Here's the drawing with two shaded views (mm, measured from the low corner). I have some questions. Round coordinates to 2 decimals unless told otherwise and drop trailing zeros. Loops run counter-clockwise (first coordinate to the right, second up) from the corner with the lowest first, then second, coordinate; pieces in that order, holes last. Notation, with made-up numbers: (16, -10) -> (24, -10) arc R19 ccw to (24, -3) -> close; hole circle Ø8 at (52.5, -30.5). An arc over 180 degrees is marked (long way). Write item = value, one per line.
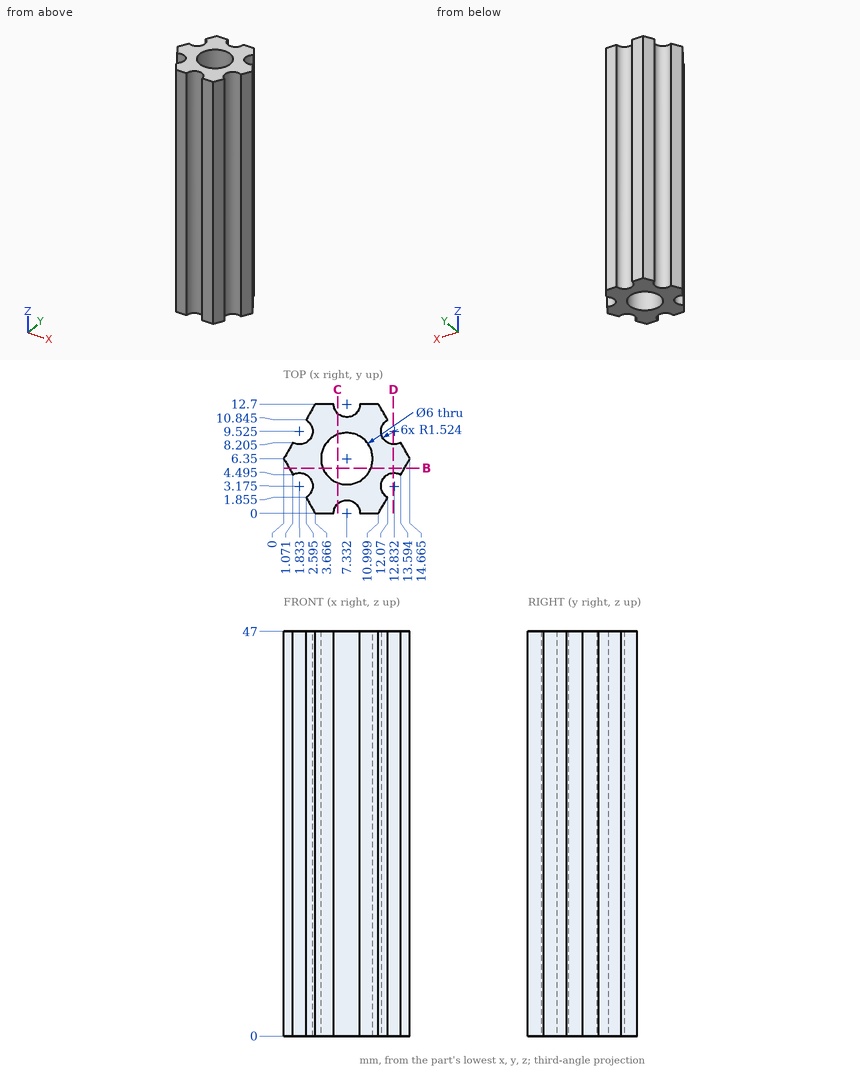
1. I need wall thicknesses on line 1 (X direction, y = 5.5, z = 23.5) (1 decimal); line 2 (Y direction, x = 6.5, z = 24) (1 decimal); line 3 (X direction, y = 7, z = 38) (1 decimal). Which ranges of each line are inside material? Lowest first, please. Write a range as [from, to].
Entries:
line_1 = [0.5, 4.5], [10.2, 14.2]
line_2 = [1.3, 3.5], [9.2, 11.4]
line_3 = [0.4, 4.4], [10.3, 14.3]
2. Suppose I cut it at B-B, the plane y = 5.25. List the corners of the cut face in (x, z) for me (1 decimal).
Entries:
outline = (0.6, 0) -> (4.5, 0) -> (4.5, 47) -> (0.6, 47) -> close; (10.1, 0) -> (14, 0) -> (14, 47) -> (10.1, 47) -> close
3. Suppose I cut it at D-D, the plane x = 12.75. List the corners of the cut face in (y, z) for me, and give its area (3 significant figures).
Entries:
outline = (4.7, 0) -> (8, 0) -> (8, 47) -> (4.7, 47) -> close
area = 155 mm²
4. I'm going to push flat-ended pins straight in: pin 1 (1 mm diameter, centred on x = 9.5, y = 7.5, fed in from +Z); pin 2 (3 mm diameter, centred on y = 9.5, z = 36, fed in from -X); pin 3 (1.5 mm diameter, centred on y = 9.5, z = 38, fed in from -X) (1 decimal). Where does each tip first touch, or does it pass through?
Entries:
pin_1 = through
pin_2 = 0.95
pin_3 = 3.1
5. Suppose I cut it at C-C, the plane x = 6.25. List the corners of the cut face in (y, z) for me.
Entries:
outline = (1.07, 0) -> (3.55, 0) -> (3.55, 47) -> (1.07, 47) -> close; (9.15, 0) -> (11.63, 0) -> (11.63, 47) -> (9.15, 47) -> close
